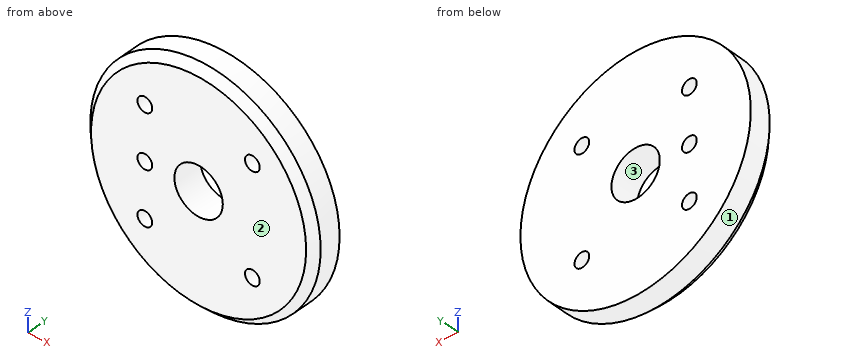
```python
from build123d import *

# Parameters (mm, degrees)
SKETCH1_R                 = 19.05
SKETCH1_R_2               = 4
BOSS_EXTRUDE1_DEPTH       = 4.7625
F_2_CLEARANCE_HOLE1_D     = 2.4384
F_2_CLEARANCE_HOLE1_DEPTH = 4.7625
CHAMFER1_SIZE             = 1.27


with BuildPart() as part:
    # Sketch1 → Boss-Extrude1 (new body)
    with BuildSketch(Plane(origin=(0, 0, 0), x_dir=(1, 0, 0), z_dir=(0, 1, 0))):
        Circle(SKETCH1_R)
        Circle(SKETCH1_R_2, mode=Mode.SUBTRACT)
    extrude(amount=BOSS_EXTRUDE1_DEPTH)

    # #2 Clearance Hole1
    with Locations(Plane(origin=(0, 4.7625, 0), x_dir=(1, 0, 0), z_dir=(0, 1, 0))):
        with Locations((-8.89, 8.89), (8.89, 8.89), (-8.89, -8.89), (8.89, -8.89), (-8.89, 0)):
            Hole(F_2_CLEARANCE_HOLE1_D / 2, depth=F_2_CLEARANCE_HOLE1_DEPTH)

    # Chamfer1
    chamfer1_edges = [part.edges().sort_by_distance(p)[0] for p in [
        (-19.05, 0, 0),
    ]]
    chamfer(chamfer1_edges, length=CHAMFER1_SIZE)


solid = part.part
```
Geometry check sheet. Reference: the model listing, model coordinates, mm. Face numbers are marked on the shaded views. Round coordinates to 2 decimals unless told otherwise and drop trailing zeros. Order: outer loops, then holes, each group sorted by start corner. A loop starts at its lowest first (then second) coordinate and runs counter-clockwise, first axis right, second up. Notation, with made-up numbers: (-39, 31) - (-5, 31) arc R22 cw to (-5, 51) - close; hole circle Ø3 at (76.5, 10). An arc over 180 degrees is marked (long way). Use a Markdown table: item, result. Add a question column.
1) Gauge pin test, flat ends, axial feed: P1, Ø1.5, axis at x = -8.89, z = -8.89, coming from the +Y side; P2, Ø2, axis at x = -15, y = 4, coming from the -Z side; P3, Ø2, axis at y = 1, z = -15, coming from the +X side. Record the tip position at first contact, or that the pin passes through.
2) Section check B-B (y = 0.7). Record the cut outline in (x, z).
3) Section check A-A (z = 0). Record the cut outline in (x, y), then the cut area to 3 significant figures.
4) Section check D-D (y = 2.75). Record the cut outline in (x, z), then the cut area to 3 significant figures.
5) Mould release check, pull along Z, two halves, no side actions. Record for the marked faces 1, 2 and 3: released by +Z, released by -Z, zero draft, split by the parting line, or undercut.
6) Thickness scan on line 1 along Z through (x, y) = (-8.89, 1.2); line 2 along X through (y, z) = (3.2, -0.5); line 3 along Z through (x, y) = (0, 1.5). Record the ranges inside material, lowest first.
7) Section check C-C (x = 0). Record the cut outline in (y, z).
Established:
| question | item | result |
|---|---|---|
| 1 | P1 | through |
| 1 | P2 | z = -12.92 |
| 1 | P3 | x = 12.88 |
| 2 | outline | circle Ø36.96 at (0, 0); hole circle Ø2.44 at (-8.89, -8.89); hole circle Ø2.44 at (-8.89, 0); hole circle Ø2.44 at (-8.89, 8.89); hole circle Ø8 at (0, 0); hole circle Ø2.44 at (8.89, -8.89); hole circle Ø2.44 at (8.89, 8.89) |
| 3 | outline | (-19.05, 1.27) - (-17.78, 0) - (-10.11, 0) - (-10.11, 4.76) - (-19.05, 4.76) - close; (-7.67, 0) - (-4, 0) - (-4, 4.76) - (-7.67, 4.76) - close; (4, 0) - (17.78, 0) - (19.05, 1.27) - (19.05, 4.76) - (4, 4.76) - close |
| 3 | area | 130 mm2 |
| 4 | outline | circle Ø38.1 at (0, 0); hole circle Ø2.44 at (-8.89, -8.89); hole circle Ø2.44 at (-8.89, 0); hole circle Ø2.44 at (-8.89, 8.89); hole circle Ø8 at (0, 0); hole circle Ø2.44 at (8.89, -8.89); hole circle Ø2.44 at (8.89, 8.89) |
| 4 | area | 1,070 mm2 |
| 5 | face 1 | split by the parting line |
| 5 | face 2 | zero draft |
| 5 | face 3 | undercut |
| 6 | line 1 | -16.77 to -10.11, -7.67 to -1.22, 1.22 to 7.67, 10.11 to 16.77 |
| 6 | line 2 | -19.04 to -10, -7.78 to -3.97, 3.97 to 19.04 |
| 6 | line 3 | -19.05 to -4, 4 to 19.05 |
| 7 | outline | (0, -17.78) - (1.27, -19.05) - (4.76, -19.05) - (4.76, -4) - (0, -4) - close; (0, 4) - (4.76, 4) - (4.76, 19.05) - (1.27, 19.05) - (0, 17.78) - close |
